from build123d import *

# Parameters (mm, degrees)
BOSS_EXTRUDE1_DEPTH = 339.725
BOSS_EXTRUDE2_REACH = 691.724
CUT_EXTRUDE4_DEPTH  = 697.975102984
SKETCH6_W           = 376.513172643
SKETCH6_H           = 53.606624692
CUT_EXTRUDE8_DEPTH  = 692.004787475
SKETCH7_W           = 213.060365226
SKETCH7_H           = 305.038721392
BOSS_EXTRUDE4_DEPTH = 5.842


with BuildPart() as part:
    # Sketch1 → Boss-Extrude1 (new body)
    with BuildSketch(Plane(origin=(0, 0, 0), x_dir=(1, 0, 0), z_dir=(0, 1, 0))):
        Polygon((0, 0), (209.55, 0), (227.063263081, 547.6875), (228.651574493, 547.6875), (211.08754833, -1.5875), (-1.53754833, -1.5875), (-19.101574493, 547.6875), (-17.513263081, 547.6875), align=None)
    extrude(amount=-BOSS_EXTRUDE1_DEPTH)

    # Boss-Extrude2: up to this plane
    boss_extrude2_end = Plane(origin=(-19.101574493, -339.725, -547.6875), z_dir=(-0.9994891356560206, 0, 0.03196040840760531))
    # Sketch3 → Boss-Extrude2 (add, up to the surface)
    with BuildSketch(Plane(origin=(210.922640445, 0, 6.744619317), x_dir=(0.031960408407605376, 0, -0.9994891356560207), z_dir=(0.9994891356560207, 0, 0.031960408407605376)), mode=Mode.PRIVATE) as boss_extrude2_sk1:
        Polygon((5.20194578, -17.461159368), (554.715503688, 0), (554.715503688, -1.588301242), (5.210173674, -19.049199163), align=None)
    boss_extrude2_tool1 = split(extrude(boss_extrude2_sk1.sketch, amount=-BOSS_EXTRUDE2_REACH, mode=Mode.PRIVATE), bisect_by=boss_extrude2_end, keep=Keep.BOTH, mode=Mode.PRIVATE)
    add(boss_extrude2_tool1.solids().sort_by_distance((219.870301, -9.524663, -273.07314))[0])
    # Sketch3 → Boss-Extrude2 (add, up to the surface)
    with BuildSketch(Plane(origin=(210.922640445, 0, 6.744619317), x_dir=(0.031960408407605376, 0, -0.9994891356560207), z_dir=(0.9994891356560207, 0, 0.031960408407605376)), mode=Mode.PRIVATE) as boss_extrude2_sk2:
        Polygon((5.159755252, -322.2625), (554.715503688, -339.725), (554.715503688, -341.313301242), (5.159755252, -323.850801242), align=None)
    boss_extrude2_tool2 = split(extrude(boss_extrude2_sk2.sketch, amount=-BOSS_EXTRUDE2_REACH, mode=Mode.PRIVATE), bisect_by=boss_extrude2_end, keep=Keep.BOTH, mode=Mode.PRIVATE)
    add(boss_extrude2_tool2.solids().sort_by_distance((219.869561, -331.787901, -273.05))[0])

    # Sketch5 → Cut-Extrude4 (cut, through all)
    with BuildSketch(Plane(origin=(210.922640445, 0, 6.744619317), x_dir=(0.031960408407605376, 0, -0.9994891356560207), z_dir=(0.9994891356560207, 0, 0.031960408407605376))):
        Polygon((5.159755252, -322.263840612), (554.715503688, -341.313301242), (-187.514814981, -341.313301242), align=None)
        Polygon((5.159755252, -17.461159388), (-85.492186458, -17.461159388), (-85.492186458, 58.963399127), (554.715503688, 0), align=None)
    extrude(amount=-CUT_EXTRUDE4_DEPTH, mode=Mode.SUBTRACT)

    # Sketch6 → Cut-Extrude8 (cut, through all)
    with BuildSketch(Plane(origin=(0, 0, 0), x_dir=(1, 0, 0), z_dir=(0, 1, 0))):
        Polygon((-1.755182613, 5.218517559), (295.768737434, 5.218517559), (295.768737434, -74.400442216), (-24.623288418, -74.400442216), align=None)
        with Locations((124.241384065, 574.490812346)):
            Rectangle(SKETCH6_W, SKETCH6_H)
    extrude(amount=-CUT_EXTRUDE8_DEPTH, mode=Mode.SUBTRACT)

    # Sketch7 → Boss-Extrude4 (add)
    with BuildSketch(Plane.XY):
        with Locations((104.775, -169.980520084)):
            Rectangle(SKETCH7_W, SKETCH7_H)
    extrude(amount=-BOSS_EXTRUDE4_DEPTH)


solid = part.part
Read the model definition and answer for the solid it produces. Units are mm, in the model's axes. Round coordinates to 2 decimals unless told otherwise and drop trailing zeros. Write each loop counter-clockwise with the first axis right and the second up, starting at its lowest first coordinate (ties: lowest second). Pieces come first, ordered by that corner, then holes.
1. The part is cut by section A-A, the plane y = -51.5. Determine the outline of the cut face in (x, z).
2. Given pin 1 Ø5 at (x, z) = (167.5, -232) entering from +Y; pin 2 Ø8 at (x, z) = (56, -462.5) entering from -Y; pin 3 Ø4.5 at (x, z) = (91.5, -3) entering from -Y, each flat-ended and moving along its own axis, determine where each tip first touches the part or whether it passes through.
3. Determine the mould class of faces 1 (the face through (103, -168, 0)), 2 (the face through (103, -169, -5.842)) for opening direction X: pulls with the +X half, pulls with the -X half, needs draft (parallel to the pull), parting line crosses it, or undercut.
4. The part is cut by section C-C, the plane x = 126.5. Determine the outline of the cut face in (y, z), then the cut area to 3 significant figures.
5. Straight lines are drawn through the part: L1, parallel to Z at x = 149, y = -22.5; L2, parallel to X at y = -93.5, z = -454; L3, parallel to X at y = -305.5, z = -387.5. For each, find the intervals that lie inside material, in ascending order.
Values:
1. outline: (-19.1, -547.69) - (-17.51, -547.69) - (-0.19, -5.84) - (209.74, -5.84) - (227.06, -547.69) - (228.65, -547.69) - (211.31, -5.22) - (211.31, 0) - (-1.76, 0) - (-1.76, -5.22) - close
2. pin 1: stops at y = -10.01
2. pin 2: stops at y = -338.31
2. pin 3: stops at y = -322.5
3. face 1: needs draft
3. face 2: undercut
4. outline: (-341.2, -547.69) - (-339.62, -547.69) - (-322.41, -5.84) - (-18.9, -5.84) - (-1.69, -547.69) - (-0.1, -547.69) - (-17.33, -5.22) - (-17.46, -5.22) - (-17.46, 0) - (-322.5, 0) - (-322.5, -5.84) - (-322.43, -5.84) - close
4. area: 3,070 mm2
5. L1: z = -5.84 to 0
5. L2: x = -16.11 to -14.52, 224.07 to 225.66
5. L3: x = -13.98 to -12.39, 221.94 to 223.53
